Can you work these out from the model? Positions are in its coordinate system, mm. Face numbers are marked on the shaded views. Give positions to 0.01 mm unless a question says otherwise; leave off trailing zeros. Order: outer loops, then holes, each group sorted by start corner. A loop starts at its lowest first (then second) coordinate and runs counter-clockwise, first axis right, second up. Notation, with made-up numbers: M 13.5,30.5 L 46.5,30.5 A23 cw 46.5,54.5 Z; hole C 81,30.5 d4. An arc over 180 degrees is marked long. Use one line per item in the form item = value. Start each with the question number.
1. I want a section at A-A, the plane y = 5. List the corners of the cut face in (x, z) for me, and give its area (3 significant figures).
2. I need wall thicknesses on L1, parallel to Y at x = 19, z = -132; L2, parallel to Z at x = 1, y = -0.5; L3, parallel to Z at x = 2, y = 14. Which ranges of each line are inside material? Lowest first, please.
3. I want a section at B-B, the plane z = -132.5. List the corners of the cut face in (x, y) for me.
4. We'd pull the mould along Y, two halves only. Please class the marked faces 1, 2 and 3: +Y half, -Y half, draft (parallel to the pull), parting line (faces both ways), or undercut.
5. I want a section at C-C, the plane x = 20.5. List the corners of the cut face in (y, z) for me.
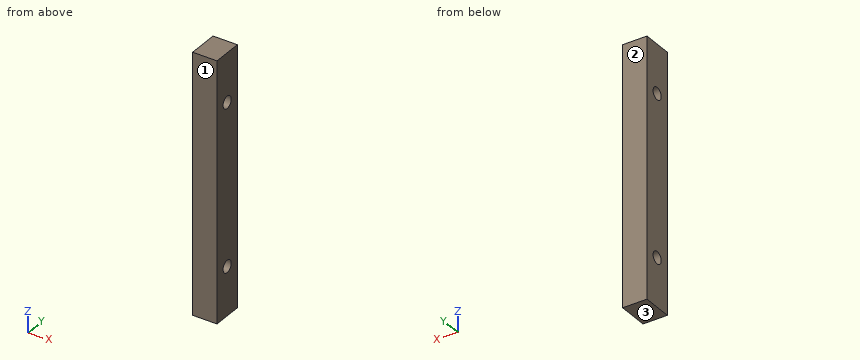
```python
from build123d import *

# Parameters (mm, degrees)
SKETCH_1_W          = 40
SKETCH_1_H          = 50
EXTRUDE_1_DEPTH     = 212.5
CUT_EXTRUDE_1_REACH = 220.303
SKETCH_2_R          = 10


with BuildPart() as part:
    # 草图1 → 凸台-拉伸1 (new, symmetric)
    with BuildSketch(Plane.XY):
        with Locations((10, 5)):
            Rectangle(SKETCH_1_W, SKETCH_1_H)
    extrude(amount=EXTRUDE_1_DEPTH, both=True)

    # 草图2 → 切除-拉伸1 (cut, up to next)
    with BuildSketch(Plane(origin=(30, 0, 0), x_dir=(0, 0, -1), z_dir=(1, 0, 0)), mode=Mode.PRIVATE) as cut_extrude_1_sk1:
        with Locations((-132.5, 5)):
            Circle(SKETCH_2_R)
    cut_extrude_1_tool1 = extrude(cut_extrude_1_sk1.sketch, amount=-CUT_EXTRUDE_1_REACH, mode=Mode.PRIVATE) & part.part
    # 草图2 → 切除-拉伸1 (cut, up to next)
    with BuildSketch(Plane(origin=(30, 0, 0), x_dir=(0, 0, -1), z_dir=(1, 0, 0)), mode=Mode.PRIVATE) as cut_extrude_1_sk2:
        with Locations((132.5, 5)):
            Circle(SKETCH_2_R)
    cut_extrude_1_tool2 = extrude(cut_extrude_1_sk2.sketch, amount=-CUT_EXTRUDE_1_REACH, mode=Mode.PRIVATE) & part.part
    add(cut_extrude_1_tool1.solids().sort_by_distance((30, 5, 132.5))[0], mode=Mode.SUBTRACT)
    add(cut_extrude_1_tool2.solids().sort_by_distance((30, 5, -132.5))[0], mode=Mode.SUBTRACT)


solid = part.part
```
Check result:
q1.outline = M -10,-212.5 L 30,-212.5 L 30,-142.5 L -10,-142.5 Z; M -10,-122.5 L 30,-122.5 L 30,122.5 L -10,122.5 Z; M -10,142.5 L 30,142.5 L 30,212.5 L -10,212.5 Z
q1.area = 15,400 mm2
q2.L1 = -20 to -4.99, 14.99 to 30
q2.L2 = -212.5 to -140.85, -124.15 to 124.15, 140.85 to 212.5
q2.L3 = -212.5 to -136.86, -128.14 to 128.14, 136.86 to 212.5
q3.outline = M -10,-20 L 30,-20 L 30,-5 L -10,-5 Z; M -10,15 L 30,15 L 30,30 L -10,30 Z
q4.face_1 = -Y half
q4.face_2 = +Y half
q4.face_3 = draft
q5.outline = M -20,-212.5 L 30,-212.5 L 30,212.5 L -20,212.5 Z; hole C 5,-132.5 d20; hole C 5,132.5 d20
